```python
from build123d import *

# Parameters (mm, degrees)
BOSS_EXTRUDE1_DEPTH     = 127
SHELL2_T                = -31.75
SKETCH2_R               = 31.75
CUT_EXTRUDE1_DEPTH      = 643.020000528
SKETCH3_R               = 31.75
CUT_EXTRUDE2_DEPTH      = 645.43437317
SKETCH4_R               = 31.75
CUT_EXTRUDE3_DEPTH      = 643.020000528
CUT_EXTRUDE4_DEPTH      = 645.43437317
CUT_EXTRUDE4_DEPTH_BACK = 645.43437317
SKETCH5_R               = 31.75


with BuildPart() as part:
    # Sketch1 → Boss-Extrude1 (new body)
    with BuildSketch(Plane(origin=(0, 0, 0), x_dir=(1, 0, 0), z_dir=(0, 1, 0))):
        Polygon((198.258990648, -190.264676509), (274.727719698, 5.652833739), (190.264676509, 198.258990648), (-5.652833739, 274.727719698), (-198.258990648, 190.264676509), (-274.727719698, -5.652833739), (-190.264676509, -198.258990648), (5.652833739, -274.727719698), align=None)
    extrude(amount=BOSS_EXTRUDE1_DEPTH)

    # Shell2
    shell2_openings = [part.faces().sort_by_distance(p)[0] for p in [
        (0, 127, 0),
    ]]
    offset(amount=SHELL2_T, openings=shell2_openings, kind=Kind.INTERSECTION)

    # Sketch2 → Cut-Extrude1 (cut, through all)
    with BuildSketch(Plane(origin=(-92.305921385, 0, 236.493355173), x_dir=(0.9315564981895357, 0, 0.36359660433074675), z_dir=(-0.36359660433074675, 0, 0.9315564981895357))):
        with Locations((-66.675, 63.5)):
            Circle(SKETCH2_R)
        with Locations((0, 63.5)):
            Circle(SKETCH2_R)
        with Locations((66.675, 63.5)):
            Circle(SKETCH2_R)
    extrude(amount=-CUT_EXTRUDE1_DEPTH, mode=Mode.SUBTRACT)

    # Sketch3 → Cut-Extrude2 (cut, through all)
    with BuildSketch(Plane(origin=(101.955912193, 0, 232.496198103), x_dir=(0.9158115414668875, 0, -0.4016082923895416), z_dir=(0.4016082923895416, 0, 0.9158115414668875))):
        with Locations((-66.802, 63.5)):
            Circle(SKETCH3_R)
        with Locations((0, 63.5)):
            Circle(SKETCH3_R)
        with Locations((66.675, 63.5)):
            Circle(SKETCH3_R)
    extrude(amount=-CUT_EXTRUDE2_DEPTH, mode=Mode.SUBTRACT)

    # Sketch4 → Cut-Extrude3 (cut, through all)
    with BuildSketch(Plane(origin=(236.493355173, 0, 92.305921385), x_dir=(0.3635966043307465, 0, -0.9315564981895359), z_dir=(0.9315564981895358, 0, 0.3635966043307464))):
        with Locations((-65.869378977, 63.5)):
            Circle(SKETCH4_R)
        with Locations((0.805621023, 63.5)):
            Circle(SKETCH4_R)
        with Locations((67.480621023, 63.5)):
            Circle(SKETCH4_R)
    extrude(amount=-CUT_EXTRUDE3_DEPTH, mode=Mode.SUBTRACT)

    # Sketch5 → Cut-Extrude4 (cut, two sides: drawn at the far end of the back side and taken through both)
    with BuildSketch(Plane(origin=(232.496198103, 0, -101.955912193), x_dir=(-0.401608292389542, 0, -0.9158115414668874), z_dir=(0.9158115414668874, 0, -0.401608292389542)).offset(-CUT_EXTRUDE4_DEPTH_BACK)):
        with Locations(Location((-66.675, 63.5, 0), (0, 0, 180))):
            Circle(SKETCH5_R)
        with Locations((0, 63.5)):
            Circle(SKETCH5_R)
        with Locations((66.675, 63.5)):
            Circle(SKETCH5_R)
    extrude(amount=CUT_EXTRUDE4_DEPTH + CUT_EXTRUDE4_DEPTH_BACK, mode=Mode.SUBTRACT)


solid = part.part
```
Geometry: final body of the model. Coordinates: model frame, mm. A direction names the side the tool comes from. Coordinates: 2 decimals unless noted, no trailing zeros. Order: outer loops, then holes, each group sorted by start corner. A loop starts at its lowest first (then second) coordinate and runs counter-clockwise, first axis right, second up. Notation, with made-up numbers: (7, -8) - (65, -8) arc R21 ccw to (65, 17) - close; hole circle Ø9 at (48, 30). An arc over 180 degrees is marked (long way). Write each question's results on one line, items separated by ' | '.
1) Line query: line 1 (Y direction, x = -160.5, z = -165); line 2 (Y direction, x = -132.5, z = 203.5); line 3 (Y direction, x = -85, z = -212). Output: solid intervals per line, ascending. Write a range as from..to.
Results list:
line 1: 0..31.75 | line 2: 0..36.84, 90.16..127 | line 3: 0..32.6, 94.4..127
2) Set-up query: faces 1 (the flat face through (160.84, 34.76, -175.66)), 2 (the cylindrical face through (208.973, 73.037, 119.765)). Return all of +Z, -Z, +X, -X, +Y, -Y with unobstructed straight access to the full face (end or side cutting, diameter ignored); none if empty.
Results list:
face 1: +Y | face 2: none
3) Section A-A, the plane y = 107.5. Return loops of the section in (x, z), plus the area to 3 significant figures.
Results list:
outline: (-274.73, 5.65) - (-198.26, -190.26) - (-5.65, -274.73) - (190.26, -198.26) - (274.73, -5.65) - (198.26, 190.26) - (5.65, 274.73) - (-190.26, 198.26) - close; hole (-240.37, 4.95) - (-173.46, -166.47) - (-4.95, -240.37) - (166.47, -173.46) - (240.37, -4.95) - (173.46, 166.47) - (4.95, 240.37) - (-166.47, 173.46) - close | area: 50,100 mm^2
4) Pin query (flat end, axial travel): pin 1 (5 mm diameter, centred on y = 79.5, z = 38.5, fed in from +X); pin 2 (10 mm diameter, centred on x = 88.5, y = 16.5, fed in from -Z); pin 3 (4 mm diameter, centred on x = -206.5, z = 16.5, fed in from +Y); pin 4 (2 mm diameter, centred on x = -19, y = 32.5, fed in from +Z). Return the tip coordinate at first contact, or that it passes through.
Results list:
pin 1: through | pin 2: z = -239.93 | pin 3: y = 31.75 | pin 4: z = 265.5
5) Pull-direction query (Y, two-part tool) for faces 3 (the cylindrical face through (-232.05, 64.9, 63.59)), 4 (the flat face through (168.94, 35.22, -167.83)), 5 (the flat face through (-3, 31.75, -3)); classes: pulls with the +Y half, pulls with the -Y half, needs draft (parallel to the pull), parting line crosses it, or undercut.
Results list:
face 3: undercut | face 4: needs draft | face 5: pulls with the +Y half
6) Section B-B, the plane z = 97.5. State how many separate pieces and enclosed holes the cut face has, plus the area to 3 significant figures.
Results list:
separate pieces: 3 | enclosed holes: 0 | area: 17,300 mm^2
